For this review, use the dimensioned drawing (mm, ordinates from the lowest corner) and the shaded views. Coordinates: 2 decimals unless noted, no trailing zeros. Write each loop counter-clockwise with the first axis right and the second up, starting at its lowest first coordinate (ties: lowest second). Pieces come first, ordered by that corner, then holes. Notation, with made-up numbers: (52, -1.75) -> (103, -1.75) arc R35 ccw to (103, 32.25) -> close; hole circle Ø10 at (63, 2.5). An arc over 180 degrees is marked (long way). Put each result on its own line as item: value. Start each with the question number.
Item 1: Consider section B-B on y = 50. Give the boundary of the cut face in (x, z), and give its area (3 significant figures).
Item 2: Consider section A-A on z = 64. Give the boundary of the cut face in (x, y).
Item 3: To check wall thickness, follow L1, parallel to Y at x = 0.75, z = 64; L2, parallel to Z at x = 0.1, y = 10.5; L3, parallel to Z at x = 0.35, y = 3.5. State the ranges of each line that lie inside material, in increasing order.
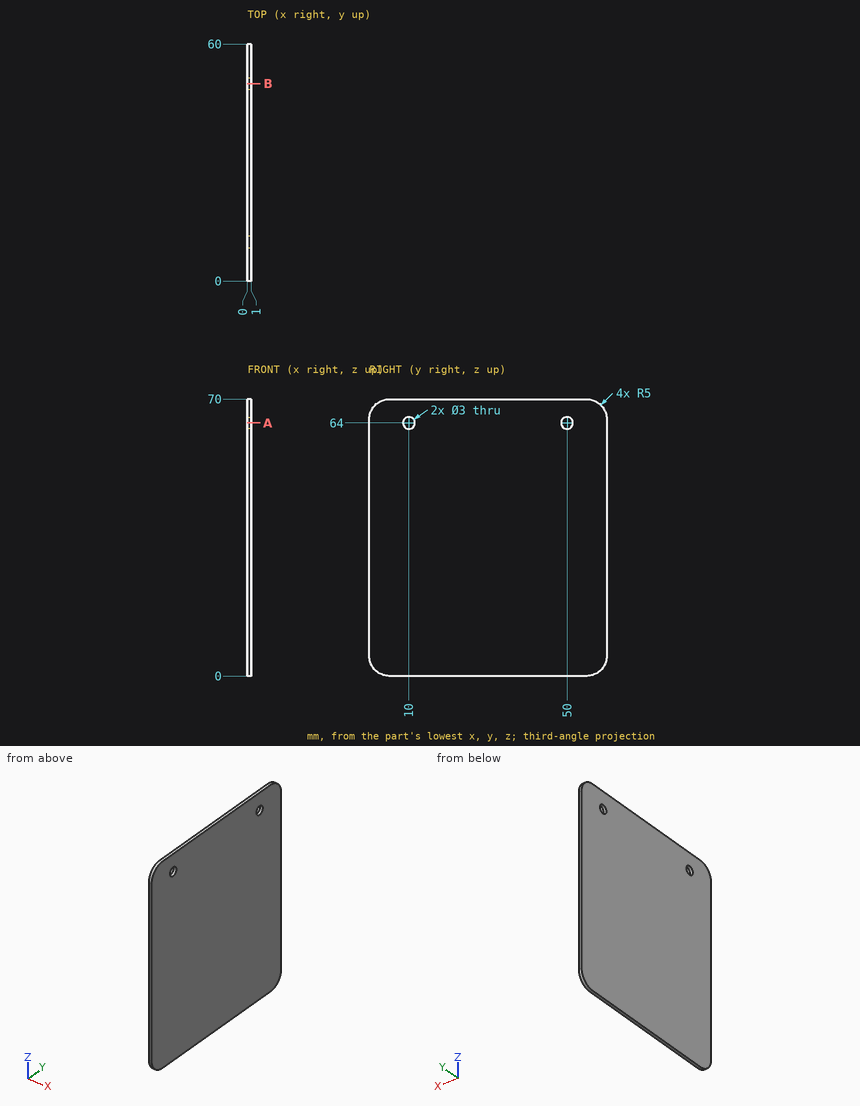
Return value:
1. outline: (0, 0) -> (1, 0) -> (1, 62.5) -> (0, 62.5) -> close; (0, 65.5) -> (1, 65.5) -> (1, 70) -> (0, 70) -> close
1. area: 67.0 mm^2
2. outline: (0, 0) -> (1, 0) -> (1, 8.5) -> (0, 8.5) -> close; (0, 11.5) -> (1, 11.5) -> (1, 48.5) -> (0, 48.5) -> close; (0, 51.5) -> (1, 51.5) -> (1, 60) -> (0, 60) -> close
3. L1: 0 to 8.5, 11.5 to 48.5, 51.5 to 60
3. L2: 0 to 62.59, 65.41 to 70
3. L3: 0.23 to 69.77
